```python
from build123d import *

# Parameters (mm, degrees)
SKETCH1_W           = 60
SKETCH1_H           = 60
BOSS_EXTRUDE1_DEPTH = 3
SKETCH2_W           = 30
SKETCH2_H           = 30
BOSS_EXTRUDE2_DEPTH = 14.999999878
SKETCH3_W           = 22
SKETCH3_H           = 22
BOSS_EXTRUDE3_DEPTH = 19.999999944
SHELL1_START        = -8
SHELL1_DEPTH        = 16
SHELL1_START_2      = -12
SHELL1_2_OUTLINE_W  = 14.999999878
SHELL1_2_OUTLINE_H  = 24
SHELL1_2_DEPTH      = 24
SKETCH4_W           = 16
SKETCH4_H           = 16
CUT_EXTRUDE1_DEPTH  = 55.999999887
SKETCH5_W           = 18
SKETCH5_H           = 18
SKETCH5_W_2         = 16
SKETCH5_H_2         = 16
CUT_EXTRUDE2_DEPTH  = 21.000000066
FILLET2_R           = 2.54
FILLET3_R           = 2.54
FILLET4_R           = 1.27


# Read off the part's stored shape, not the designer's step: Shell1
with BuildPart() as part:
    # Sketch1 → Boss-Extrude1 (new body)
    with BuildSketch(Plane(origin=(0, 0, 0), x_dir=(1, 0, 0), z_dir=(0, 1, 0))):
        Rectangle(SKETCH1_W, SKETCH1_H)
    extrude(amount=BOSS_EXTRUDE1_DEPTH)

    # Sketch2 → Boss-Extrude2 (add)
    with BuildSketch(Plane(origin=(0, 3, 0), x_dir=(1, 0, 0), z_dir=(0, 1, 0))):
        Rectangle(SKETCH2_W, SKETCH2_H)
    extrude(amount=BOSS_EXTRUDE2_DEPTH)

    # Sketch3 → Boss-Extrude3 (add)
    with BuildSketch(Plane(origin=(0, 17.999999878, 0), x_dir=(1, 0, 0), z_dir=(0, 1, 0))):
        Rectangle(SKETCH3_W, SKETCH3_H)
    extrude(amount=BOSS_EXTRUDE3_DEPTH)

    # Shell1 outline → Shell1 (cut)
    with BuildSketch(Plane.YZ.offset(SHELL1_START)):
        Polygon((14.999999878, 12), (0, 12), (0, -12), (14.999999878, -12), (14.999999878, -8), (34.999999822, -8), (34.999999822, 8), (14.999999878, 8), align=None)
    extrude(amount=SHELL1_DEPTH, mode=Mode.SUBTRACT)

    # Shell1 2 outline → Shell1 2 (cut)
    with BuildSketch(Plane.YZ.offset(SHELL1_START_2)):
        with Locations((7.499999939, 0)):
            Rectangle(SHELL1_2_OUTLINE_W, SHELL1_2_OUTLINE_H)
    extrude(amount=SHELL1_2_DEPTH, mode=Mode.SUBTRACT)

    # Sketch4 → Cut-Extrude1 (cut, through all)
    with BuildSketch(Plane.XZ.offset(-34.999999822)):
        Rectangle(SKETCH4_W, SKETCH4_H)
    extrude(amount=-CUT_EXTRUDE1_DEPTH, mode=Mode.SUBTRACT)

    # Sketch5 → Cut-Extrude2 (cut)
    with BuildSketch(Plane(origin=(0, 37.999999822, 0), x_dir=(1, 0, 0), z_dir=(0, 1, 0))):
        Rectangle(SKETCH5_W, SKETCH5_H)
        Rectangle(SKETCH5_W_2, SKETCH5_H_2, mode=Mode.SUBTRACT)
    extrude(amount=-CUT_EXTRUDE2_DEPTH, mode=Mode.SUBTRACT)

    # Fillet2
    fillet2_edges = [part.edges().sort_by_distance(p)[0] for p in [
        (-12, 0, 0),
        (-12, 7.499999939, -12),
        (0, 0, 12),
        (-12, 7.499999939, 12),
        (12, 0, 0),
        (12, 7.499999939, 12),
        (0, 0, -12),
        (12, 7.499999939, -12),
        (-12, 14.999999878, 0),
        (0, 14.999999878, 12),
        (12, 14.999999878, 0),
        (0, 14.999999878, -12),
    ]]
    fillet(fillet2_edges, radius=FILLET2_R)

    # Fillet3
    fillet3_edges = [part.edges().sort_by_distance(p)[0] for p in [
        (-15, 10.499999939, -15),
        (-15, 10.499999939, 15),
        (15, 10.499999939, 15),
        (15, 10.499999939, -15),
        (-11, 27.99999985, -11),
        (-11, 27.99999985, 11),
        (11, 27.99999985, 11),
        (11, 27.99999985, -11),
        (-30, 1.5, -30),
        (30, 1.5, -30),
        (30, 1.5, 30),
        (-30, 1.5, 30),
    ]]
    fillet(fillet3_edges, radius=FILLET3_R)
    fillet3_2_edges = [part.edges().sort_by_distance(p)[0] for p in [
        (-15, 3, 0),
        (0, 3, 15),
        (15, 3, 0),
        (0, 3, -15),
        (-11, 17.999999878, 0),
        (0, 17.999999878, 11),
        (11, 17.999999878, 0),
        (0, 17.999999878, -11),
        (10.256051224, 17.999999878, -10.256051224),
        (-10.256051224, 17.999999878, -10.256051224),
        (10.256051224, 17.999999878, 10.256051224),
        (-10.256051224, 17.999999878, 10.256051224),
        (-14.256051224, 3, -14.256051224),
        (14.256051224, 3, -14.256051224),
        (14.256051224, 3, 14.256051224),
        (-14.256051224, 3, 14.256051224),
    ]]
    fillet(fillet3_2_edges, radius=FILLET3_R)

    # Fillet4
    fillet4_edges = [part.edges().sort_by_distance(p)[0] for p in [
        (-15, 17.999999878, 0),
        (0, 17.999999878, 15),
        (15, 17.999999878, 0),
        (0, 17.999999878, -15),
        (-14.256051224, 17.999999878, -14.256051224),
        (-14.256051224, 17.999999878, 14.256051224),
        (14.256051224, 17.999999878, 14.256051224),
        (14.256051224, 17.999999878, -14.256051224),
    ]]
    fillet(fillet4_edges, radius=FILLET4_R)


solid = part.part
```
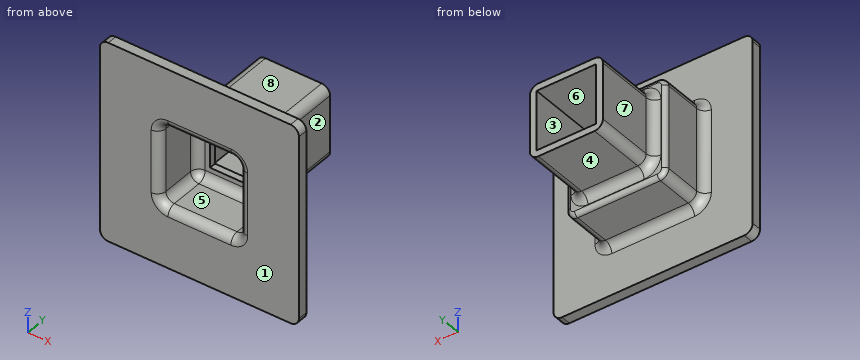
Input: part model. Units: mm. Frame: model coordinates. Face numbers are marked on the shaded views. A direction names the side the tool comes from. Coordinates: 2 decimals unless noted, no trailing zeros. Write each loop counter-clockwise with the first axis right and the second up, starting at its lowest first coordinate (ties: lowest second). Pieces come first, ordered by that corner, then holes. Notation, with made-up numbers: (-5.75, -31) -> (-1.75, -31) arc R25 cw to (-1.75, -13) -> close; hole circle Ø1 at (-23, -22). An arc over 180 degrees is marked (long way). Answer as a JSON object with one key per item and string values.
1. Material intervals for line 1 (X direction, y = 7, z = 6); line 2 (X direction, y = 25, z = -4), sorted ascending. Write a range as from..to.
Result set:
{"line 1": "x = -15..-12, 12..15", "line 2": "x = -11..-9, 9..11"}
2. Section D-D on z = -21. Return the cut outline in (x, y).
Result set:
{"outline": "(-30, 0) -> (30, 0) -> (30, 3) -> (-30, 3) -> close"}
3. Mould query, pull axis X, two halves, no side actions, for the marked faces 1, 2 and 3. Classes: released by +X, released by -X, zero draft, split by the parting line, or undercut.
Result set:
{"face 1": "zero draft", "face 2": "released by +X", "face 3": "undercut"}
4. Access query for the marked faces 4, 5, 6, 7 and 8. Directions: +Z, -Z, +X, -X, +Y, -Y. A direction counts if a zero-diameter tool reaches every point of the face in a straight line with its end or side. Return the directions, or none.
Result set:
{"face 4": "-Z, +X, -X, +Y", "face 5": "-Y", "face 6": "+Y", "face 7": "+Z, -Z, -X, +Y", "face 8": "+Z, +X, -X, +Y"}
5. First-contact query: P1, Ø5.5, axis at y = 31, z = -3, coming from the +X side; P2, Ø8.5, axis at y = 33.5, z = 3, coming from the -X side; P3, Ø6, axis at x = 12.5, z = 7.5, coming from the -Y side; P4, Ø1.6, axis at x = 2, y = 16, coming from the -Z side. Flat tips, straight axial feed; report the tip coordinate or a pass-through.
Result set:
{"P1": "stops at x = 11", "P2": "stops at x = -11", "P3": "stops at y = 0", "P4": "stops at z = -15"}
6. Section C-C on y = 28.5. Return the cut outline in (x, z), then the cut area to 3 significant figures.
Result set:
{"outline": "(-11, -8.46) arc R2.54 ccw to (-8.46, -11) -> (8.46, -11) arc R2.54 ccw to (11, -8.46) -> (11, 8.46) arc R2.54 ccw to (8.46, 11) -> (-8.46, 11) arc R2.54 ccw to (-11, 8.46) -> close; hole (-9, -9) -> (9, -9) -> (9, 9) -> (-9, 9) -> close", "area": "154 mm2"}
